```python
from build123d import *

# Parameters (mm, degrees)
BOSS_EXTRUDE1_DEPTH     = 6
CUT_EXTRUDE1_DEPTH      = 35.525353003
CUT_EXTRUDE1_DEPTH_BACK = 35.525353003
FILLET1_R               = 2
FILLET2_R               = 1
FILLET3_R               = 0.811424
FILLET4_R               = 2
FILLET5_R               = 1
FILLET6_R               = 1
FILLET7_R               = 0.5
FILLET8_R               = 0.6
SKETCH4_R               = 1.5
CUT_EXTRUDE2_DEPTH      = 8.5


with BuildPart() as part:
    # Sketch2 → Boss-Extrude1 (new, symmetric)
    with BuildSketch(Plane.XY):
        Polygon((6.5, 11), (-6.5, 11), (-8, 4.9838286), (-8, 0), (-12.25, 0), (-12.25, 3.981133366), (-10.5, 11), (-15, 11), (-15, 13), (-17, 13), (-17, 6), (-17.75, 6), (-17.75, 5), (-17, 4.813003998), (-17, 3.813003998), (-18.387819958, 0), (-24.387819958, 0), (-30, 1.50377911), (-30, 5.00377911), (-28.5, 5.00377911), (-28.5, 3.172407682), (-26.2783706, 2.577123878), (-28.785442178, 11.933642386), (-30, 12.5), (-30, 16), (0, 16), (30, 16), (30, 8), (21.339745962, 3), (17.839745962, 3), (15.4, 3.608296988), (15.4, 4.214079193), (17.75, 4.8), (17.75, 6), (12.35, 6), (12.35, 11), (10.5, 11), (12.25, 3.981133366), (12.25, 0), (8, 0), (8, 4.9838286), align=None)
    extrude(amount=BOSS_EXTRUDE1_DEPTH, both=True)

    # Sketch3 → Cut-Extrude1 (cut, two sides: drawn at the far end of the back side and taken through both)
    with BuildSketch(Plane.XY.offset(-CUT_EXTRUDE1_DEPTH_BACK)):
        Polygon((-27.626331186, 12.24422524), (-24.667039952, 1.2), (-19.228069004, 1.2), (-18.249764702, 3.88786898), (-18.95, 4.062457248), (-18.95, 7.2), (-18.2, 7.2), (-18.2, 13), (-20.2, 13), (-20.2, 2.2), (-23.899712964, 2.2), (-26.66040536, 12.503044285), align=None)
        Polygon((13.55, 11), (13.55, 7.2), (18.95, 7.2), (18.95, 4.2), (21.018206931, 4.2), (28.8, 8.692820323), (28.8, 11), align=None)
    extrude(amount=CUT_EXTRUDE1_DEPTH + CUT_EXTRUDE1_DEPTH_BACK, mode=Mode.SUBTRACT)

    # Fillet1
    fillet1_edges = [part.edges().sort_by_distance(p)[0] for p in [
        (12.35, 6, 0),
    ]]
    fillet(fillet1_edges, radius=FILLET1_R)

    # Fillet2
    fillet2_edges = [part.edges().sort_by_distance(p)[0] for p in [
        (13.55, 7.2, 0),
    ]]
    fillet(fillet2_edges, radius=FILLET2_R)

    # Fillet3
    fillet3_edges = [part.edges().sort_by_distance(p)[0] for p in [
        (12.35, 11, 0),
        (10.5, 11, 0),
    ]]
    fillet(fillet3_edges, radius=FILLET3_R)

    # Fillet4
    fillet4_edges = [part.edges().sort_by_distance(p)[0] for p in [
        (12.25, 3.981133366, 0),
        (8, 4.9838286, 0),
        (6.5, 11, 0),
        (-6.5, 11, 0),
        (-8, 4.9838286, 0),
        (-12.25, 3.981133366, 0),
    ]]
    fillet(fillet4_edges, radius=FILLET4_R)

    # Fillet5
    fillet5_edges = [part.edges().sort_by_distance(p)[0] for p in [
        (-20.2, 13, 0),
        (-18.2, 13, 0),
    ]]
    fillet(fillet5_edges, radius=FILLET5_R - 0.0001)  # a hair under: the kernel refuses the full size

    # Fillet6
    fillet6_edges = [part.edges().sort_by_distance(p)[0] for p in [
        (-15, 13, 0),
        (-17, 13, 0),
    ]]
    fillet(fillet6_edges, radius=FILLET6_R - 0.0001)  # a hair under: the kernel refuses the full size

    # Fillet7
    fillet7_edges = [part.edges().sort_by_distance(p)[0] for p in [
        (-27.626331186, 12.24422524, 0),
        (-26.66040536, 12.503044285, 0),
    ]]
    fillet(fillet7_edges, radius=FILLET7_R - 0.0001)  # a hair under: the kernel refuses the full size

    # Fillet8
    fillet8_edges = [part.edges().sort_by_distance(p)[0] for p in [
        (-23.899712964, 2.2, 0),
        (-20.2, 2.2, 0),
        (-19.228069004, 1.2, 0),
        (-24.667039952, 1.2, 0),
        (13.55, 11, 0),
        (28.8, 11, 0),
        (28.8, 8.692820323, 0),
        (18.95, 4.2, 0),
        (18.95, 7.2, 0),
        (12.25, 0, 0),
        (8, 0, 0),
        (-8, 0, 0),
        (-12.25, 0, 0),
        (-10.5, 11, 0),
        (-15, 11, 0),
        (-18.387819958, 0, 0),
        (-24.387819958, 0, 0),
        (-30, 1.50377911, 0),
        (-28.5, 3.172407682, 0),
        (-26.2783706, 2.577123878, 0),
        (-28.785442178, 11.933642386, 0),
        (-30, 12.5, 0),
        (30, 8, 0),
        (21.339745962, 3, 0),
        (17.839745962, 3, 0),
    ]]
    fillet(fillet8_edges, radius=FILLET8_R)

    # Sketch4 → Cut-Extrude2 (cut)
    with BuildSketch(Plane(origin=(0, 16, 0), x_dir=(1, 0, 0), z_dir=(0, 1, 0))):
        with Locations(Location((-23, 0, 0), (0, 0, 270))):
            Circle(SKETCH4_R)
        with Locations(Location((23, 0, 0), (0, 0, 180))):
            Circle(SKETCH4_R)
    extrude(amount=-CUT_EXTRUDE2_DEPTH, mode=Mode.SUBTRACT)


solid = part.part
```
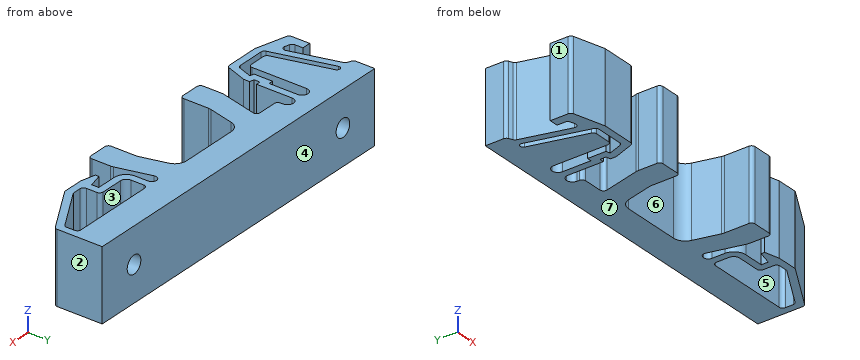
Geometry check sheet. Reference: the model listing, model coordinates, mm. Face numbers are marked on the shaded views. A direction names the side the tool comes from. Give positions to 0.01 mm unless a question says otherwise; leave off trailing zeros. Loops run counter-clockwise (first coordinate to the right, second up) from the corner with the lowest first, then second, coordinate; pieces in that order, holes last. Notation, with made-up numbers: M 74.5,-29 L 113.5,-29 A11 ccw 113.5,-25 Z; hole C -0.5,-15.5 d7. An arc over 180 degrees is marked long. Answer as CSV lines item,"result".
Item 1: Material ranges on line 1 (Y direction, x = 17.5, z = 5.75); line 2 (X direction, y = 11.25, z = 3.5); line 3 (Z direction, x = 23, y = 13.4), recorded low to high.
Values:
line 1,"y = 3.08 to 4.74, 6 to 7.2, 11 to 16"
line 2,"x = -28.6 to -27.36, -26.32 to -20.2, -18.2 to -17, -14.89 to 30"
line 3,"z = -6 to -1.5, 1.5 to 6"
Item 2: Release check for a two-part mould opening along X. For the marked faces 1, 2, 3 and 4 record: pulls with the +X half, pulls with the -X half, needs draft (parallel to the pull), parting line crosses it, or undercut.
Values:
face 1,"pulls with the -X half"
face 2,"pulls with the +X half"
face 3,"undercut"
face 4,"needs draft"
Item 3: Cross-section at B-B on z = 2.75. Count the separate pieces of the cut face and the enclosed holes in it, and give its area (3 significant figures).
Values:
separate pieces,"1"
enclosed holes,"2"
area,"505 mm²"
Item 4: Access from +Z, -Z, +X, -X, +Y, -Y to the whole of each face (thin tool, end or side, straight path). Record for the marked faces 5, 6 and 7.
Values:
face 5,"+Z, -Z"
face 6,"+Z, -Z, -Y"
face 7,"-Z, +X, -X, +Y, -Y"
Item 5: Depth check by flat-ended pin: P1, Ø6, axis at x = 4, y = 6, coming from the +Z side; P2, Ø1.8, axis at x = 23, z = 0, coming from the -Y side; P3, Ø3, axis at x = -0.5, z = 0.5, coming from the -Y side; P4, Ø0.5, axis at y = 5.5, z = -2, coming from the +X side. Enter the tip coordinate at first touch or a pass-through.
Values:
P1,"passes through"
P2,"stops at y = 3.44"
P3,"stops at y = 11"
P4,"stops at x = 26.1"
Item 6: Cross-section at A-A on x = 23. Record the cut outline in (y, z).
Values:
outline,"M 3.96,-6 L 5.34,-6 L 5.34,6 L 3.96,6 Z; M 11,-6 L 16,-6 L 16,-1.5 L 11,-1.5 Z; M 11,1.5 L 16,1.5 L 16,6 L 11,6 Z"
